from build123d import *

# Parameters (mm, degrees)
SKETCH1_W           = 790
SKETCH1_H           = 80
BOSS_EXTRUDE1_DEPTH = 6
SKETCH2_W           = 6
SKETCH2_H           = 25
SKETCH2_H_2         = 15
CUT_EXTRUDE1_DEPTH  = 6
SKETCH3_W           = 30
SKETCH3_H           = 6
BOSS_EXTRUDE2_DEPTH = 6


with BuildPart() as part:
    # Sketch1 → Boss-Extrude1 (new body)
    with BuildSketch(Plane.XY):
        Rectangle(SKETCH1_W, SKETCH1_H)
    extrude(amount=BOSS_EXTRUDE1_DEPTH)

    # Sketch2 → Cut-Extrude1 (cut)
    with BuildSketch(Plane(origin=(0, 0, 0), x_dir=(-1, 0, 0), z_dir=(0, 0, -1))):
        with Locations((392, 27.5)):
            Rectangle(SKETCH2_W, SKETCH2_H)
        with Locations((392, -27.5)):
            Rectangle(SKETCH2_W, SKETCH2_H)
        with Locations((-392, -27.5)):
            Rectangle(SKETCH2_W, SKETCH2_H)
        with Locations((-392, 27.5)):
            Rectangle(SKETCH2_W, SKETCH2_H)
        with Locations((66, -22.5)):
            Rectangle(SKETCH2_W, SKETCH2_H_2)
        with Locations((182, -22.5)):
            Rectangle(SKETCH2_W, SKETCH2_H_2)
        with Locations((182, 22.5)):
            Rectangle(SKETCH2_W, SKETCH2_H_2)
        with Locations((66, 22.5)):
            Rectangle(SKETCH2_W, SKETCH2_H_2)
        with Locations((-50, -22.5)):
            Rectangle(SKETCH2_W, SKETCH2_H_2)
        with Locations((-50, 22.5)):
            Rectangle(SKETCH2_W, SKETCH2_H_2)
        with Locations((-166, -22.5)):
            Rectangle(SKETCH2_W, SKETCH2_H_2)
        with Locations((-166, 22.5)):
            Rectangle(SKETCH2_W, SKETCH2_H_2)
        with Locations((-282, -22.5)):
            Rectangle(SKETCH2_W, SKETCH2_H_2)
        with Locations((-282, 22.5)):
            Rectangle(SKETCH2_W, SKETCH2_H_2)
    extrude(amount=-CUT_EXTRUDE1_DEPTH, mode=Mode.SUBTRACT)

    # Sketch3 → Boss-Extrude2 (add)
    with BuildSketch(Plane(origin=(0, 0, 0), x_dir=(-1, 0, 0), z_dir=(0, 0, -1))):
        with Locations((-30, -43)):
            Rectangle(SKETCH3_W, SKETCH3_H)
        with Locations((-30, 43)):
            Rectangle(SKETCH3_W, SKETCH3_H)
        with Locations((-110, -43)):
            Rectangle(SKETCH3_W, SKETCH3_H)
        with Locations((-110, 43)):
            Rectangle(SKETCH3_W, SKETCH3_H)
        with Locations((-190, -43)):
            Rectangle(SKETCH3_W, SKETCH3_H)
        with Locations((-190, 43)):
            Rectangle(SKETCH3_W, SKETCH3_H)
        with Locations((-270, -43)):
            Rectangle(SKETCH3_W, SKETCH3_H)
        with Locations((-270, 43)):
            Rectangle(SKETCH3_W, SKETCH3_H)
        with Locations((-350, -43)):
            Rectangle(SKETCH3_W, SKETCH3_H)
        with Locations((-350, 43)):
            Rectangle(SKETCH3_W, SKETCH3_H)
        with Locations((350, 43)):
            Rectangle(SKETCH3_W, SKETCH3_H)
        with Locations((350, -43)):
            Rectangle(SKETCH3_W, SKETCH3_H)
        with Locations((270, 43)):
            Rectangle(SKETCH3_W, SKETCH3_H)
        with Locations((270, -43)):
            Rectangle(SKETCH3_W, SKETCH3_H)
        with Locations((190, 43)):
            Rectangle(SKETCH3_W, SKETCH3_H)
        with Locations((190, -43)):
            Rectangle(SKETCH3_W, SKETCH3_H)
        with Locations((110, 43)):
            Rectangle(SKETCH3_W, SKETCH3_H)
        with Locations((110, -43)):
            Rectangle(SKETCH3_W, SKETCH3_H)
        with Locations((30, 43)):
            Rectangle(SKETCH3_W, SKETCH3_H)
        with Locations((30, -43)):
            Rectangle(SKETCH3_W, SKETCH3_H)
    extrude(amount=-BOSS_EXTRUDE2_DEPTH)


solid = part.part
Input: part model. Units: mm. Frame: model coordinates. Coordinates: 2 decimals unless noted, no trailing zeros. Loops run counter-clockwise (first coordinate to the right, second up) from the corner with the lowest first, then second, coordinate; pieces in that order, holes last.
Q1. Cut plane A-A (x = 299). Output: boundary loops of the cut face in (y, z), then the cut area to 3 significant figures.
Q2. Contact query for flat-ended pins moving along their axis: pin 1 (1.8 mm diameter, centred on x = -392, z = 1.5, fed in from -Y); pin 2 (3 mm diameter, centred on x = -66.5, z = 3.5, fed in from -Y); pin 3 (3 mm diameter, centred on y = 20, z = 1.5, fed in from -X). Output: stop coordinate, or through.
Q3. Material intervals for line 1 (X direction, y = -17, z = 4.35); line 2 (Y direction, x = 212.5, z = 1.3); line 3 (X direction, y = -32, z = 3.85), sorted ascending.
Q4. Cut plane B-B (z = 2.1). Give the number of separate pieces and of enclosed holes in the cut face, then the cut area to 3 significant figures.
Working result:
1. outline: (-40, 0) - (40, 0) - (40, 6) - (-40, 6) - close
1. area: 480 mm2
2. pin 1: stops at y = -15
2. pin 2: stops at y = -40
2. pin 3: stops at x = -389
3. line 1: x = -389 to -185, -179 to -69, -63 to 47, 53 to 163, 169 to 279, 285 to 389
3. line 2: y = -40 to 40
3. line 3: x = -389 to 389
4. separate pieces: 1
4. enclosed holes: 10
4. area: 65,300 mm2
